Source: CAD feature listing. Evaluate the final solid. Frame: model axes, mm. Give positions to 0.01 mm unless a question says otherwise; leave off trailing zeros. Order: outer loops, then holes, each group sorted by start corner. A loop starts at its lowest first (then second) coordinate and runs counter-clockwise, first axis right, second up.
1) Material intervals for line 1 (X direction, y = 1, z = 1); line 2 (Y direction, x = 172.5, z = -2.75); line 3 (X direction, y = -3, z = -2), sorted ascending.
2) Section A-A, the plane y = 0. Return loops of the section in (x, z), plus the area to 3 significant figures.
3) First-contact query: P1, Ø11.5, axis at x = 172.5, y = 0, coming from the +Z side. Flat tip, straight axial feed; report the tip coordinate or a pass-through.
4) Section B-B, the plane x = 77.5. Return loops of the section in (y, z).
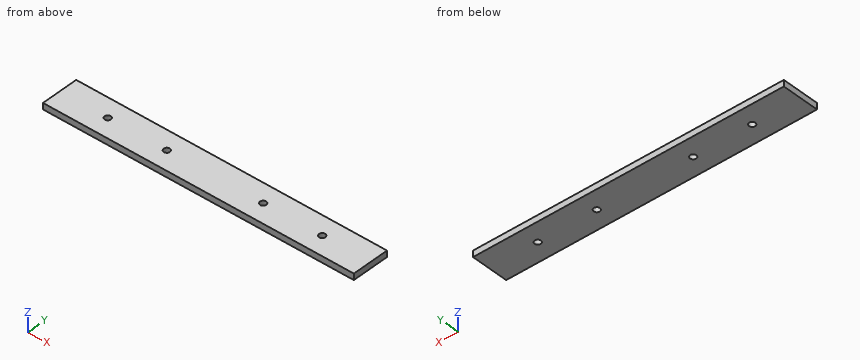
```python
from build123d import *

# Parameters (mm, degrees)
SKETCH1_W           = 500
SKETCH1_H           = 60
SKETCH1_R           = 5
BOSS_EXTRUDE1_DEPTH = 5


with BuildPart() as part:
    # Sketch1 → Boss-Extrude1 (new, symmetric)
    with BuildSketch(Plane.XY):
        Rectangle(SKETCH1_W, SKETCH1_H)
        with Locations((172.5, 0)):
            Circle(SKETCH1_R, mode=Mode.SUBTRACT)
        with Locations((77.5, 0)):
            Circle(SKETCH1_R, mode=Mode.SUBTRACT)
        with Locations(Location((-172.5, 0, 0), (0, 0, 180))):
            Circle(SKETCH1_R, mode=Mode.SUBTRACT)
        with Locations(Location((-77.5, 0, 0), (0, 0, 180))):
            Circle(SKETCH1_R, mode=Mode.SUBTRACT)
    extrude(amount=BOSS_EXTRUDE1_DEPTH, both=True)


solid = part.part
```
From the geometry:
1. line 1: x = -250 to -177.4, -167.6 to -82.4, -72.6 to 72.6, 82.4 to 167.6, 177.4 to 250
1. line 2: y = -30 to -5, 5 to 30
1. line 3: x = -250 to -176.5, -168.5 to -81.5, -73.5 to 73.5, 81.5 to 168.5, 176.5 to 250
2. outline: (-250, -5) - (-177.5, -5) - (-177.5, 5) - (-250, 5) - close; (-167.5, -5) - (-82.5, -5) - (-82.5, 5) - (-167.5, 5) - close; (-72.5, -5) - (72.5, -5) - (72.5, 5) - (-72.5, 5) - close; (82.5, -5) - (167.5, -5) - (167.5, 5) - (82.5, 5) - close; (177.5, -5) - (250, -5) - (250, 5) - (177.5, 5) - close
2. area: 4,600 mm2
3. P1: stops at z = 5
4. outline: (-30, -5) - (-5, -5) - (-5, 5) - (-30, 5) - close; (5, -5) - (30, -5) - (30, 5) - (5, 5) - close
